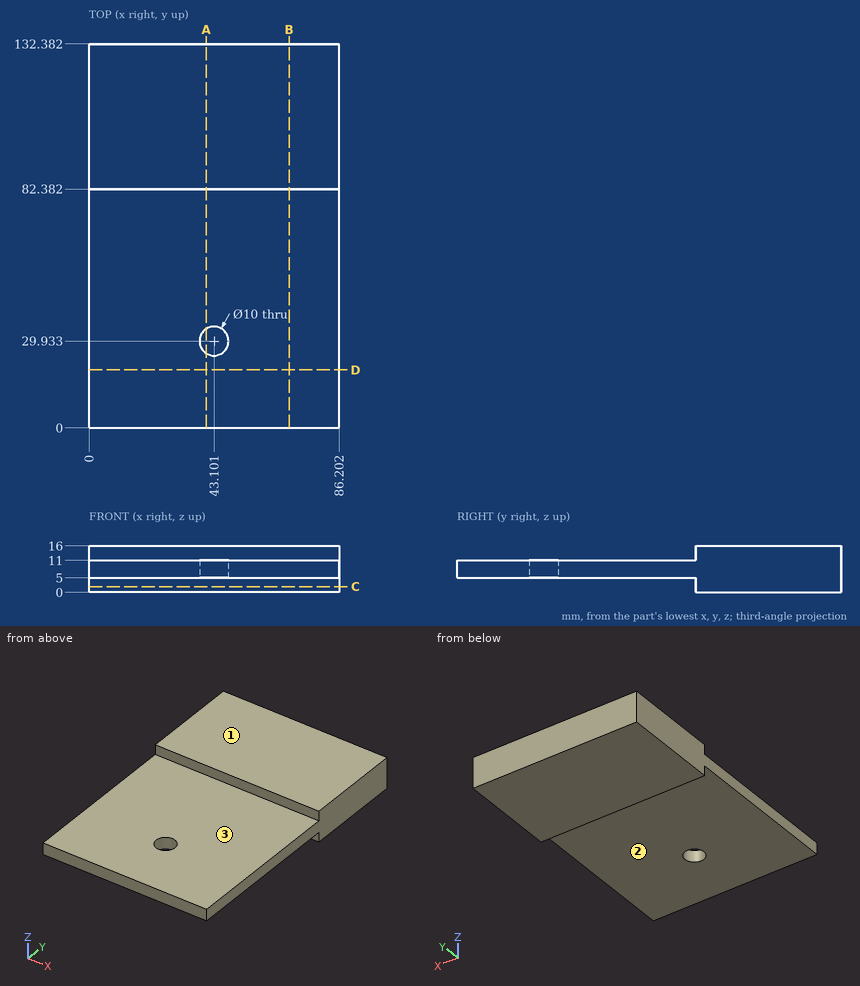
Geometry: see drawing. Coordinates: mm, zero at the bounding-box minimum. A direction names the side the tool comes from. Round coordinates to 2 decimals unless told otherwise and drop trailing zeros. Loops run counter-clockwise (first coordinate to the right, second up) from the corner with the lowest first, then second, coordinate; pieces in that order, holes last. Notation, with made-up numbers: (59, 9) -> (111, 9) arc R12 ccw to (111, 15) -> close; hole circle Ø3 at (-38, -0.75). An arc over 180 degrees is marked (long way). One line per question, with ' | ' between items. Start each with the question number.
1. Section B-B on x = 69. Output: boundary loops of the cut face in (y, z), and give its area (3 significant figures).
2. Set-up query: the marked faces 1, 2 and 3. Return all of +Z, -Z, +X, -X, +Y, -Y with unobstructed straight access to the full face (end or side cutting, diameter ignored); none if empty.
3. Section A-A on x = 40.5. Output: boundary loops of the cut face in (y, z).
4. Contact query for flat-ended pins moving along their axis: pin 1 (3 mm diameter, centred on x = 21.5, z = 2, fed in from -Y); pin 2 (24.5 mm diameter, centred on x = 56.5, y = 43.5, fed in from -Z). Output: stop coordinate, or through.
5. Line query: line 1 along Z through (x, y) = (11, 75.5); line 2 along Y through (x, z) = (40, 2.25). Output: solid intervals per line, ascending. Write a range as [from, to].
6. Section C-C on z = 2. Output: boundary loops of the cut face in (x, y), and give its area (3 significant figures).
7. Section D-D on y = 20. Output: boundary loops of the cut face in (x, z), and give its area (3 significant figures).
Returned:
1) outline: (0, 5) -> (82.38, 5) -> (82.38, 0) -> (132.38, 0) -> (132.38, 16) -> (82.38, 16) -> (82.38, 11) -> (0, 11) -> close | area: 1,290 mm2
2) face 1: +Z, +X, -X, +Y, -Y | face 2: -Z, +X, -X, -Y | face 3: +Z, +X, -X, -Y
3) outline: (0, 5) -> (25.66, 5) -> (25.66, 11) -> (0, 11) -> close; (34.2, 5) -> (82.38, 5) -> (82.38, 0) -> (132.38, 0) -> (132.38, 16) -> (82.38, 16) -> (82.38, 11) -> (34.2, 11) -> close
4) pin 1: stops at y = 82.38 | pin 2: stops at z = 5
5) line 1: z = [5, 11] | line 2: y = [82.38, 132.38]
6) outline: (0, 82.38) -> (86.2, 82.38) -> (86.2, 132.38) -> (0, 132.38) -> close | area: 4,310 mm2
7) outline: (0, 5) -> (86.2, 5) -> (86.2, 11) -> (0, 11) -> close | area: 517 mm2
